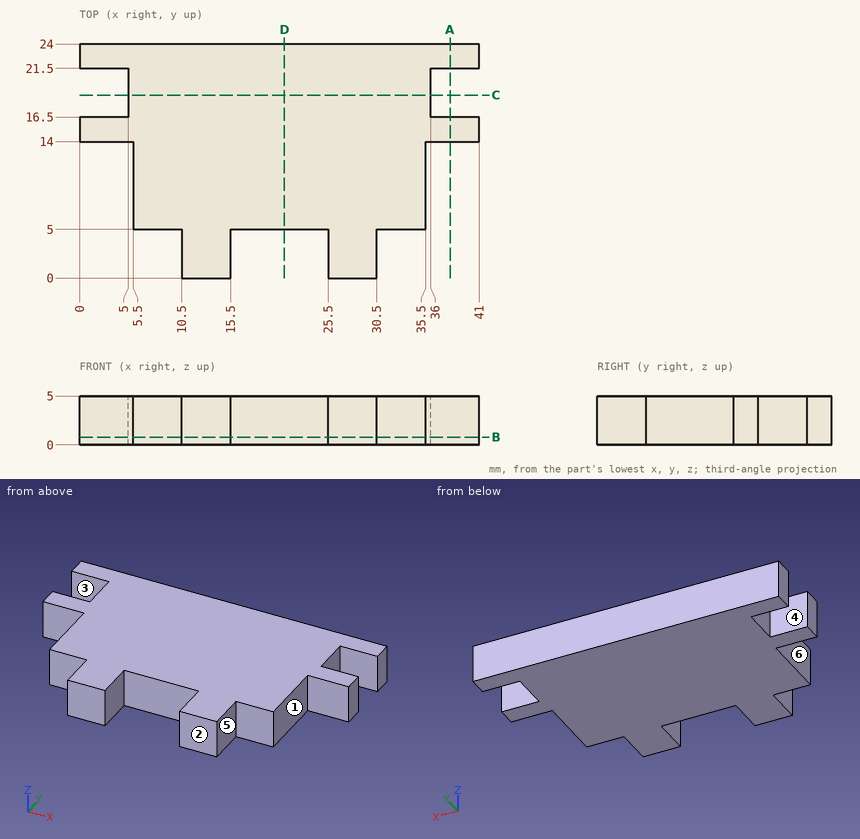
The figure shows three views and two pictorial views of one solid part (mm, origin at its lowest corner). Answer the questions. A direction names the side the tool comes from. Round coordinates to 2 decimals unless told otherwise and drop trailing zeros. Write each loop counter-clockwise with the first axis right and the second up, starting at its lowest first coordinate (ties: lowest second). Pieces come first, ordered by that corner, then holes. Notation, with made-up numbers: (-23.75, -29.75) -> (-2.75, -29.75) arc R23 ccw to (-2.75, -1.75) -> close; hole circle Ø7 at (-30.5, 13). An arc over 180 degrees is marked (long way). Write each question's results on one line, items separated by ' | '.
Q1. Straight lines are drawn through the part: line 1 along Y through (x, z) = (39, 3.7); line 2 along X through (y, z) = (1, 3.1); line 3 along Y through (x, z) = (17, 1.45). For each, find the intervals that lie inside material, in ascending order. Write a range as [from, to].
Data:
line 1: [14, 16.5], [21.5, 24] | line 2: [10.5, 15.5], [25.5, 30.5] | line 3: [5, 24]
Q2. Section D-D, the plane x = 21 is taken. Write down the section's boundary in (y, z), then the cut area to 3 significant figures.
Data:
outline: (5, 0) -> (24, 0) -> (24, 5) -> (5, 5) -> close | area: 95.0 mm^2
Q3. Section A-A, the plane x = 38 is taken. Write down the section's boundary in (y, z).
Data:
outline: (14, 0) -> (16.5, 0) -> (16.5, 5) -> (14, 5) -> close; (21.5, 0) -> (24, 0) -> (24, 5) -> (21.5, 5) -> close
Q4. Which of the six approach directions +Z, -Z, +X, -X, +Y, -Y give full straight-line access (tool end or side, diameter ignored) to the marked faces 4, 5 and 6?
Data:
face 4: +Z, -Z, -X | face 5: +Z, -Z, +X, -Y | face 6: +Z, -Z, -X, -Y
Q5. Section B-B, the plane z = 0.8 is taken. Write down the section's boundary in (x, y).
Data:
outline: (0, 14) -> (5.5, 14) -> (5.5, 5) -> (10.5, 5) -> (10.5, 0) -> (15.5, 0) -> (15.5, 5) -> (25.5, 5) -> (25.5, 0) -> (30.5, 0) -> (30.5, 5) -> (35.5, 5) -> (35.5, 14) -> (41, 14) -> (41, 16.5) -> (36, 16.5) -> (36, 21.5) -> (41, 21.5) -> (41, 24) -> (0, 24) -> (0, 21.5) -> (5, 21.5) -> (5, 16.5) -> (0, 16.5) -> close
Q6. Flat-ended cylindrical pins translate along their axes: P1, Ø2.5, axis at x = 3, z = 3.5, coming from the -Y side; P2, Ø1.5, axis at y = 18, z = 2.5, coming from the +X side; P3, Ø1.5, axis at y = 18, z = 3, coming from the -X side. Find the tip coordinate at first contact, or state that the pin passes through.
Data:
P1: y = 14 | P2: x = 36 | P3: x = 5
Q7. Determine the mould class of the marked faces 1, 2 and 3 for opening direction Y: released by +Y, released by -Y, zero draft, split by the parting line, or undercut.
Data:
face 1: zero draft | face 2: released by -Y | face 3: undercut
Q8. Section C-C, the plane y = 18.75 is taken. Write down the section's boundary in (x, z).
Data:
outline: (5, 0) -> (36, 0) -> (36, 5) -> (5, 5) -> close
